Source: CAD feature listing. Evaluate the final solid. Frame: model axes, mm. Face numbers are marked on the shaded views. A direction names the side the tool comes from. Round coordinates to 2 decimals unless told otherwise and drop trailing zeros. Loops run counter-clockwise (first coordinate to the right, second up) from the corner with the lowest first, then second, coordinate; pieces in that order, holes last.
Item 1: Section query A-A on x = 50. Return loops of the section in (y, z).
Item 2: Section query C-C on y = -8. Return loops of the section in (x, z), then the cut area to 3 significant figures.
Item 3: First-contact query: P1, Ø1, axis at x = 26.5, y = 15, coming from the -Z side; P2, Ø12, axis at y = 17, z = 42.5, coming from the -X side; P3, Ø1.5, axis at y = -1.5, z = 43.5, coming from the -X side. Flat tips, straight axial feed; report the tip coordinate or a pass-through.
Item 4: Pull-direction query (X, two-part tool) for the marked faces 5, 6 and 7; classes: released by +X, released by -X, zero draft, split by the parting line, or undercut.
Item 5: Section query D-D on z = 65.5. Return loops of the section in (x, y), then the cut area to 3 significant figures.
Item 6: Section query B-B on z = 40. Return loops of the section in (x, y), then the cut area to 3 significant figures.
Item 7: Access query for the marked faces 1, 2, 3 and 4. Directions: +Z, -Z, +X, -X, +Y, -Y. A direction counts if a zero-diameter tool reaches every point of the face in a straight line with its end or side. Return the directions, or none.
Item 8: Ray query, L1, parallel to Z at x = 50, y = -3.5; L2, parallel to X at y = 8, z = 40; L3, parallel to X at y = -13, z = 40. Return the intervals inside material, ascending.
```python
from build123d import *

# Parameters (mm, degrees)
BOSS_EXTRUDE1_DEPTH      = 10
BOSS_EXTRUDE1_DEPTH_BACK = 10
SKETCH2_W                = 50
SKETCH2_H                = 30
BOSS_EXTRUDE2_DEPTH      = 25
BOSS_EXTRUDE2_DEPTH_BACK = 25
SKETCH3_R                = 6
CUT_EXTRUDE1_DEPTH       = 51


with BuildPart() as part:
    # Sketch1 → Boss-Extrude1 (new body, two sides)
    with BuildSketch(Plane(origin=(0, 0, 0), x_dir=(1, 0, 0), z_dir=(0, 1, 0))) as boss_extrude1_sk:
        Polygon((0, 0), (30, 0), (30, -10), (70, -10), (70, 0), (100, 0), (100, -30), (85, -30), (85, -50), (100, -50), (100, -80), (70, -80), (70, -70), (30, -70), (30, -80), (0, -80), (0, -50), (15, -50), (15, -30), (0, -30), align=None)
    extrude(amount=BOSS_EXTRUDE1_DEPTH)
    extrude(boss_extrude1_sk.sketch, amount=-BOSS_EXTRUDE1_DEPTH_BACK)

    # Sketch2 → Boss-Extrude2 (add, two sides)
    with BuildSketch(Plane(origin=(0, 0, 0), x_dir=(1, 0, 0), z_dir=(0, 1, 0))) as boss_extrude2_sk:
        with Locations((50, -40)):
            Rectangle(SKETCH2_W, SKETCH2_H)
    extrude(amount=BOSS_EXTRUDE2_DEPTH)
    extrude(boss_extrude2_sk.sketch, amount=-BOSS_EXTRUDE2_DEPTH_BACK)

    # Sketch3 → Cut-Extrude1 (cut, through all)
    with BuildSketch(Plane(origin=(0, 25, 0), x_dir=(1, 0, 0), z_dir=(0, 1, 0))):
        with Locations((50, -40)):
            Circle(SKETCH3_R)
    extrude(amount=-CUT_EXTRUDE1_DEPTH, mode=Mode.SUBTRACT)


solid = part.part
```
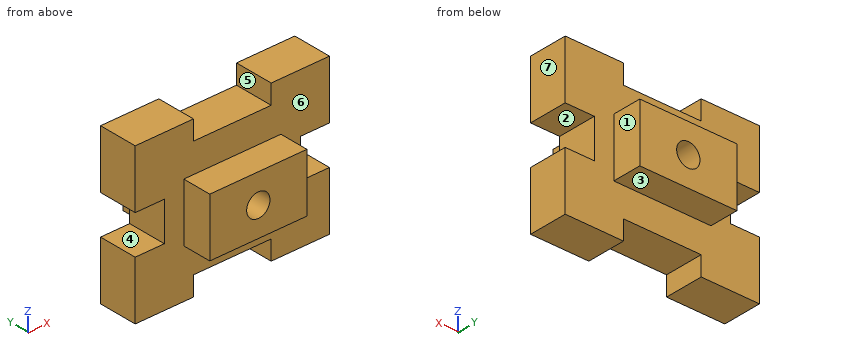
Data:
1. outline: (-25, 25) - (-10, 25) - (-10, 10) - (10, 10) - (10, 25) - (25, 25) - (25, 34) - (-25, 34) - close; (-25, 46) - (25, 46) - (25, 55) - (10, 55) - (10, 70) - (-10, 70) - (-10, 55) - (-25, 55) - close
2. outline: (0, 0) - (30, 0) - (30, 10) - (70, 10) - (70, 0) - (100, 0) - (100, 30) - (85, 30) - (85, 50) - (100, 50) - (100, 80) - (70, 80) - (70, 70) - (30, 70) - (30, 80) - (0, 80) - (0, 50) - (15, 50) - (15, 30) - (0, 30) - close; hole circle Ø12 at (50, 40)
2. area: 6,490 mm2
3. P1: stops at z = 25
3. P2: stops at x = 25
3. P3: stops at x = 15
4. face 5: undercut
4. face 6: zero draft
4. face 7: released by +X
5. outline: (0, -10) - (100, -10) - (100, 10) - (0, 10) - close
5. area: 2,000 mm2
6. outline: (15, -10) - (25, -10) - (25, -25) - (44, -25) - (44, 25) - (25, 25) - (25, 10) - (15, 10) - close; (56, -25) - (75, -25) - (75, -10) - (85, -10) - (85, 10) - (75, 10) - (75, 25) - (56, 25) - close
6. area: 2,300 mm2
7. face 1: +Z, -Z, +X, +Y
7. face 2: +X, +Y, -Y
7. face 3: -Z, +X, -X, +Y
7. face 4: -X, +Y, -Y
8. L1: z = 10 to 34, 46 to 70
8. L2: x = 15 to 44, 56 to 85
8. L3: x = 25 to 44, 56 to 75
